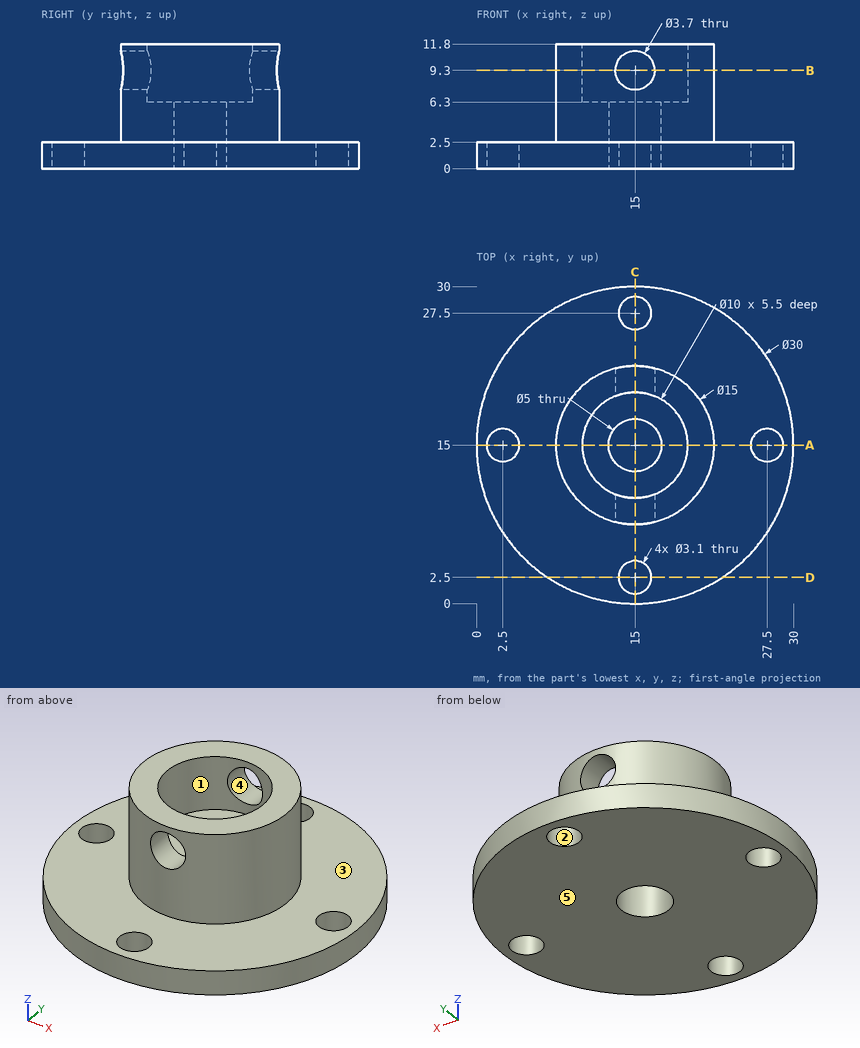
Verification items for this drawing (mm, ordinates from the low corner). A direction names the side the tool comes from. Give positions to 0.01 mm unless a question says otherwise; leave off trailing zeros. Order: outer loops, then holes, each group sorted by start corner. A loop starts at its lowest first (then second) coordinate and runs counter-clockwise, first axis right, second up. Notation, with made-up numbers: M 79,86.25 L 138,86.25 A31 ccw 138,111.25 Z; hole C 46,61 d8. An arc over 180 degrees is marked long. Use a Markdown table: item, result.
Item 1: Draft check along Z on the marked faces 3, 4 and 5. Enter one of: +Z half, -Z half, draft (parallel to the pull), parting line (faces both ways), or undercut.
Answers follow:
| item | result |
|---|---|
| face 3 | +Z half |
| face 4 | undercut |
| face 5 | -Z half |
Item 2: Depth check by flat-ended pin: P1, Ø6, axis at x = 15, z = 9.3, coming from the -Y side; P2, Ø1, axis at x = 3.5, y = 17, coming from the -Z side; P3, Ø2, axis at y = 12, z = 8.5, coming from the -X side; P4, Ø6, axis at y = 19, z = 9, coming from the -X side. Enter the tip coordinate at first touch or a pass-through.
Answers follow:
| item | result |
|---|---|
| P1 | stops at y = 7.5 |
| P2 | stops at z = 0 |
| P3 | stops at x = 7.77 |
| P4 | stops at x = 7.57 |
Item 3: Section check D-D (y = 2.5). Record the cut outline in (x, z).
Answers follow:
| item | result |
|---|---|
| outline | M 6.71,0 L 13.45,0 L 13.45,2.5 L 6.71,2.5 Z; M 16.55,0 L 23.29,0 L 23.29,2.5 L 16.55,2.5 Z |
Item 4: Section check C-C (x = 15). State how many separate pieces and enclosed holes the cut face has, and give its area (3 significant figures).
Answers follow:
| item | result |
|---|---|
| separate pieces | 6 |
| enclosed holes | 0 |
| area | 94.0 mm2 |
Item 5: Tool access check on the marked faces 1 and 2. Record the directions out of +Z, -Z, +X, -X, +Y, -Y that give a thin tool (end or side, any length) a straight path to the whole face; none if there is none.
Answers follow:
| item | result |
|---|---|
| face 1 | +Z |
| face 2 | +Z, -Z |
Item 6: Section check A-A (y = 15). Record the cut outline in (x, z), and give its area (4 significant figures).
Answers follow:
| item | result |
|---|---|
| outline | M 0,0 L 0.95,0 L 0.95,2.5 L 0,2.5 Z; M 4.05,0 L 12.5,0 L 12.5,6.3 L 10,6.3 L 10,11.8 L 7.5,11.8 L 7.5,2.5 L 4.05,2.5 Z; M 17.5,0 L 25.95,0 L 25.95,2.5 L 22.5,2.5 L 22.5,11.8 L 20,11.8 L 20,6.3 L 17.5,6.3 Z; M 29.05,0 L 30,0 L 30,2.5 L 29.05,2.5 Z |
| area | 112.5 mm2 |
Item 7: Material ranges on line 1 along Y through (x, z) = (15, 1.1); line 2 along Z through (x, y) = (15, 8.9); line 3 along Z through (x, y) = (19.5, 8.25), recorded low to high.
Answers follow:
| item | result |
|---|---|
| line 1 | y = 0 to 0.95, 4.05 to 12.5, 17.5 to 25.95, 29.05 to 30 |
| line 2 | z = 0 to 7.45, 11.15 to 11.8 |
| line 3 | z = 0 to 2.5 |
Item 8: Section check B-B (z = 9.3). Record the cut outline in (x, y), and give its area (3 significant figures).
Answers follow:
| item | result |
|---|---|
| outline | M 13.15,7.73 L 13.15,10.35 A5 cw 13.15,19.65 L 13.15,22.27 A7.5 ccw Z; M 16.85,7.73 A7.5 ccw 16.85,22.27 L 16.85,19.65 A5 cw 16.85,10.35 Z |
| area | 79.4 mm2 |
